```python
from build123d import *

# Parameters (mm, degrees)
F0_W     = 1219.2
F0_H     = 71.835716
F0_H_2   = 50.8
F1_DEPTH = 50.8
F3_R     = 3.175
F2_R     = 3.175
F4_DEPTH = 25.4
F0_W_2   = 50.8
F0_H_3   = 152.4
F5_DEPTH = 50.8


with BuildPart() as f1:
    # F0 (on Front) → F1 (new body)
    with BuildSketch(Plane.XZ):
        Polygon((1206.330058, 2246.750314), (1155.530058, 2246.750314), (1155.530058, 2174.914598), (1155.530058, -39.249686), (1155.530058, -90.049686), (1206.330058, -90.049686), align=None)
        with Locations((545.930058, 2210.832456)):
            Rectangle(F0_W, F0_H)
        Polygon((-63.669942, 2246.750314), (-114.469942, 2246.750314), (-114.469942, -90.049686), (-63.669942, -90.049686), (-63.669942, -39.249686), (-63.669942, 2174.914598), align=None)
        with Locations((545.930058, -64.649686)):
            Rectangle(F0_W, F0_H_2)
    extrude(amount=F1_DEPTH)

    # F3 (on face) + F2 (on face) → F4 (join)
    with BuildSketch(Plane.XZ.offset(50.8)):
        with Locations((-95.419942, 1691.125314)):
            Circle(F3_R)
        with Locations((-95.419942, 1735.575314)):
            Circle(F3_R)
    with BuildSketch(Plane.XZ.offset(50.8)):
        with Locations((-95.419942, 1735.575314)):
            Circle(F2_R)
    extrude(amount=F4_DEPTH)

    # F0 (on Front) → F5 (join)
    with BuildSketch(Plane.XZ):
        Polygon((1206.330058, 2246.750314), (1155.530058, 2246.750314), (1155.530058, 2174.914598), (1155.530058, -39.249686), (1155.530058, -90.049686), (1206.330058, -90.049686), align=None)
        with Locations((1180.930058, -166.249686)):
            Rectangle(F0_W_2, F0_H_3)
        with Locations((-89.069942, -166.249686)):
            Rectangle(F0_W_2, F0_H_3)
    extrude(amount=F5_DEPTH)


solid = f1.part
```
Check sheet for the modelled part. Datum: model origin and axes. Units: mm. A direction names the side the tool comes from. Round coordinates to 2 decimals unless told otherwise and drop trailing zeros. Order: outer loops, then holes, each group sorted by start corner. A loop starts at its lowest first (then second) coordinate and runs counter-clockwise, first axis right, second up. Notation, with made-up numbers: (75, 18) -> (118, 18) arc R25 ccw to (118, 41) -> close; hole circle Ø5 at (44, -13). An arc over 180 degrees is marked (long way). Use CSV: the item, a comma, the result in double quotes.
(1) Draft check along X on faces 4 (the face through (537, -25, -90.05)), 5 (the face through (-114.47, -25, 1020)), 6 (the face through (-93, -50.8, 1377)), 7 (the face through (1206.33, -25, 985)). Enter one of: pulls with the +X half, pulls with the -X half, needs draft (parallel to the pull), parting line crosses it, or undercut.
Worked out:
face 4,"undercut"
face 5,"pulls with the -X half"
face 6,"needs draft"
face 7,"pulls with the +X half"
(2) Material ranges on line 1 along Z through (x, y) = (1151.5, -13.5); line 2 along X through (y, z) = (-48.5, 2029.5), recorded low to high. Write a range as from..to.
Worked out:
line 1,"-90.05..-39.25, 2174.91..2246.75"
line 2,"-114.47..-63.67, 1155.53..1206.33"
(3) Cross-section at C-C (z = 711.5). Record the boundary of the cut face in (x, y).
Worked out:
outline,"(-114.47, -50.8) -> (-63.67, -50.8) -> (-63.67, 0) -> (-114.47, 0) -> close; (1155.53, -50.8) -> (1206.33, -50.8) -> (1206.33, 0) -> (1155.53, 0) -> close"
(4) Tool access check on faces 1 (the face through (-63.67, -25, -167)), 2 (the face through (537, -25, -39.25)), 3 (the face through (1181, -25, -242.45)). Record the directions out of +Z, -Z, +X, -X, +Y, -Y that give a thin tool (end or side, any length) a straight path to the whole face; none if there is none.
Worked out:
face 1,"-Z, +Y, -Y"
face 2,"+Y, -Y"
face 3,"-Z, +X, -X, +Y, -Y"
(5) Depth check by flat-ended pin: pin 1 (15 mm diameter, centred on x = 569, y = -33.5, fed in from -Z). Enter the tip coordinate at first touch or a pass-through.
Worked out:
pin 1,"z = -90.05"
(6) Cross-section at B-B (y = -16.5). Record the boundary of the cut face in (x, z).
Worked out:
outline,"(-114.47, -242.45) -> (-63.67, -242.45) -> (-63.67, -90.05) -> (1155.53, -90.05) -> (1155.53, -242.45) -> (1206.33, -242.45) -> (1206.33, 2246.75) -> (-114.47, 2246.75) -> close; hole (-63.67, -39.25) -> (1155.53, -39.25) -> (1155.53, 2174.91) -> (-63.67, 2174.91) -> close"
(7) Cross-section at A-A (x = 785.5). Record the boundary of the cut face in (y, z), and give its area (3 significant figures).
Worked out:
outline,"(-50.8, -90.05) -> (0, -90.05) -> (0, -39.25) -> (-50.8, -39.25) -> close; (-50.8, 2174.91) -> (0, 2174.91) -> (0, 2246.75) -> (-50.8, 2246.75) -> close"
area,"6,230 mm²"
